Autodesk Inventor part; units mm, degrees
ref_plane "YZ Plane" through (0, 0, 0) normal (1, 0, 0) x (0, 1, 0)
ref_plane "XZ Plane" through (0, 0, 0) normal (0, 1, 0) x (-1, 0, 0)
ref_plane "XY Plane" through (0, 0, 0) normal (0, 0, 1) x (1, 0, 0)
sketch "Sketch1" plane through (0, 0, 0) normal (0, 1, 0) x (-1, 0, 0)
  circle A0 centre (0, 0) radius 14.25
  dimension "d0" = 28.5
extrude "Extrusion1" add sketch "Sketch1" along normal blind 5
sketch "Sketch2" plane through (0, 5, 0) normal (0, 1, 0) x (1, 0, 0)
  circle A0 centre (0, 0) radius 14.25
  circle A1 centre (0, 0) radius 7.9
  dimension "d3" = 15.8
extrude "Extrusion2" add sketch "Sketch2" along normal blind 20 contours A1
sketch "Sketch3" plane through (0, 25, 0) normal (0, 1, 0) x (1, 0, 0)
  circle A0 centre (0, 0) radius 7.9
  circle A1 centre (0, 0) radius 5
  dimension "d6" = 10
extrude "Extrusion3" cut sketch "Sketch3" against normal blind 25.6 contours A1
chamfer "Chamfer1" distance 0.5 angle 45 1 edges at (-7.9, 25, 0)
chamfer "Chamfer2" distance 0.5 angle 45 3 edges at (-7.9, 5, 0) (14.25, 5, 0) (14.25, 0, 0)
thread "Thread1"
sketch "Sketch4" plane through (0, 0, 0) normal (0, -1, 0) x (1, 0, 0)
  circle A0 centre (0, 0) radius 13.75
  line L0 (0, 0) -> (0, -13.75) construction
  line L1 (0, 0) -> (-11.9078, 6.875) construction
  line L2 (0, 0) -> (11.9078, 6.875) construction
  circle A1 centre (0, 0) radius 14.25
  circle A2 centre (0, 0) radius 11.25 construction
  circle A3 centre (9.7428, 5.625) radius 1.5
  circle A4 centre (0, -11.25) radius 1.5
  circle A5 centre (-9.7428, 5.625) radius 1.5
  dimension "d17" = 120
  dimension "d18" = 120
  dimension "d22" = 22.5
  dimension "d23" = 3
  dimension "d24" = 3
  dimension "d25" = 3
extrude "Extrusion4" cut sketch "Sketch4" against normal blind 5 contours A3 | A4 | A5
properties part number "ZACMENut" material "ABS Plastic"
Verification items for the finished model (mm, model axes). A direction names the side the tool comes from. Coordinates: 2 decimals unless noted, no trailing zeros. Loops run counter-clockwise (first coordinate to the right, second up) from the corner with the lowest first, then second, coordinate; pieces in that order, holes last. Notation, with made-up numbers: (-37.5, 82) -> (-30.5, 82) arc R23 cw to (-30.5, 112) -> close; hole circle Ø2 at (65, 43.5). An arc over 180 degrees is marked (long way). Put each result on its own line as item: value.
1. Section check C-C, the plane y = 15.75. Record the boundary of the cut face in (x, z).
Result set:
outline: circle Ø15.8 at (0, 0); hole circle Ø10 at (0, 0)
2. Tool access check on faces 1 (the face through (6.3, 5, -5.9)), 2 (the face through (-1.08, 12.68, 4.88)). Record the directions out of +Z, -Z, +X, -X, +Y, -Y that give a thin tool (end or side, any length) a straight path to the whole face; none if there is none.
Result set:
face 1: +Y
face 2: +Y, -Y
3. Section check B-B, the plane z = 0. Record the boundary of the cut face in (x, y).
Result set:
outline: (-14.25, 0.5) -> (-13.75, 0) -> (-5, 0) -> (-5, 25) -> (-7.4, 25) -> (-7.9, 24.5) -> (-7.9, 5.5) -> (-8.4, 5) -> (-13.75, 5) -> (-14.25, 4.5) -> close; (5, 0) -> (13.75, 0) -> (14.25, 0.5) -> (14.25, 4.5) -> (13.75, 5) -> (8.4, 5) -> (7.9, 5.5) -> (7.9, 24.5) -> (7.4, 25) -> (5, 25) -> close
4. Section check A-A, the plane x = 0. Record the boundary of the cut face in (y, z), then the cut area to 3 significant figures.
Result set:
outline: (0, -13.75) -> (0.5, -14.25) -> (4.5, -14.25) -> (5, -13.75) -> (5, -12.75) -> (0, -12.75) -> close; (0, -9.75) -> (5, -9.75) -> (5, -8.4) -> (5.5, -7.9) -> (24.5, -7.9) -> (25, -7.4) -> (25, -5) -> (0, -5) -> close; (0, 5) -> (25, 5) -> (25, 7.4) -> (24.5, 7.9) -> (5.5, 7.9) -> (5, 8.4) -> (5, 13.75) -> (4.5, 14.25) -> (0.5, 14.25) -> (0, 13.75) -> close
area: 193 mm^2
5. Section check D-D, the plane y = 3. Record the boundary of the cut face in (x, z) (3 decimals), then the cut area to 3 significant figures.
Result set:
outline: circle Ø28.5 at (0, 0); hole circle Ø3 at (-9.743, 5.625); hole circle Ø10 at (0, 0); hole circle Ø3 at (0, -11.25); hole circle Ø3 at (9.743, 5.625)
area: 538 mm^2
6. Thickness scan on line 1 (X direction, y = 3.75, z = -0.25); line 2 (Z direction, x = 0, y = 3.25); line 3 (X direction, y = 7.5, z = 0). Record the ranges inside material, lowest first.
Result set:
line 1: x = -14.25 to -4.99, 4.99 to 14.25
line 2: z = -14.25 to -12.75, -9.75 to -5, 5 to 14.25
line 3: x = -7.9 to -5, 5 to 7.9
7. Gauge pin test, flat ends, axial feed: P1, Ø4, axis at y = 14.5, z = 6.5, coming from the +X side; P2, Ø6, axis at x = 11, z = -8, coming from the +Y side; P3, Ø8, axis at x = 7, y = 4, coming from the +Z side. Record the tip position at first contact, or that the pin passes through.
Result set:
P1: stops at x = 6.49
P2: stops at y = 5
P3: stops at z = 13.93
8. Mould release check, pull along Z, two halves, no side actions. Record for faces 3 (the face through (-0.325, 2.465, -12.714)), 4 (the face through (0, 0, -6)), 5 (the face through (-6.269, 14.867, -4.807)): pulls with the +Z half, pulls with the -Z half, needs draft (parallel to the pull), parting line crosses it, or undercut.
Result set:
face 3: undercut
face 4: needs draft
face 5: parting line crosses it
